Can you work these out from the drawing? Everything is in mm from the part's minimum corner. A direction names the side the tool comes from. Give positions to 0.01 mm unless a question says otherwise; leave off trailing zeros. Write each loop counter-clockwise with the first axis right and the second up, starting at its lowest first coordinate (ties: lowest second). Pieces come first, ordered by that corner, then holes. Notation, with made-up numbers: (89, -8) - (135, -8) arc R21 ccw to (135, 18) - close; hole circle Ø6 at (47.25, 7.25). An arc over 180 degrees is marked (long way). Answer in a Markdown table with one row per item.
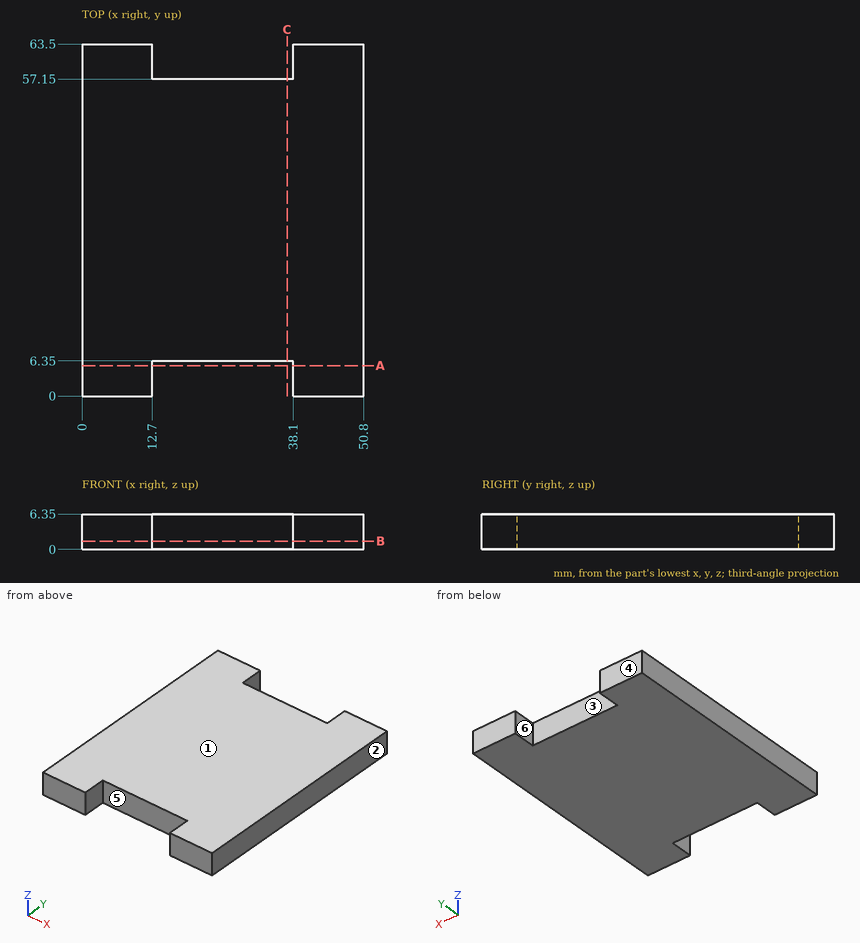
1) We'd pull the mould along X, two halves only. Please class the marked faces 1, 2 and 3: +X half, -X half, draft (parallel to the pull), parting line (faces both ways), or undercut.
Check values:
| item | result |
|---|---|
| face 1 | draft |
| face 2 | +X half |
| face 3 | undercut |
2) Will these pins go through, and if not, where does the flat tip stop? P1, Ø3, axis at x = 33.5, z = 4.5, coming from the +Y side; P2, Ø3, axis at x = 30.5, z = 3.5, coming from the -Y side.
Check values:
| item | result |
|---|---|
| P1 | stops at y = 57.15 |
| P2 | stops at y = 6.35 |
3) Imagine slicing it at A-A (y = 5.5). List the corners of the cut face in (x, z) for me, then the cut area to 3 significant figures.
Check values:
| item | result |
|---|---|
| outline | (0, 0) - (12.7, 0) - (12.7, 6.35) - (0, 6.35) - close; (38.1, 0) - (50.8, 0) - (50.8, 6.35) - (38.1, 6.35) - close |
| area | 161 mm2 |
4) If I drill on line 1 (X direction, y = 59, z = 1); line 2 (Y direction, x = 38, z = 1), over which ranges is the centre line in solid material (lowest first)?
Check values:
| item | result |
|---|---|
| line 1 | x = 0 to 12.7, 38.1 to 50.8 |
| line 2 | y = 6.35 to 57.15 |
5) Imagine slicing it at C-C (x = 37). List the corners of the cut face in (y, z) for me.
Check values:
| item | result |
|---|---|
| outline | (6.35, 0) - (57.15, 0) - (57.15, 6.35) - (6.35, 6.35) - close |
6) On a 3-axis mill with a long thin cutter (end or side, diameter ignored), from which of +Z, -Z, +X, -X, +Y, -Y can I reach the whole of each face in a straight line? I mean the marked faces 4, 5 and 6. Say none if no direction works.
Check values:
| item | result |
|---|---|
| face 4 | +Z, -Z, +X, -X, +Y |
| face 5 | +Z, -Z, -Y |
| face 6 | +Z, -Z, +Y |
7) Imagine slicing it at B-B (z = 1.5). List the corners of the cut face in (x, y) for me.
Check values:
| item | result |
|---|---|
| outline | (0, 0) - (12.7, 0) - (12.7, 6.35) - (38.1, 6.35) - (38.1, 0) - (50.8, 0) - (50.8, 63.5) - (38.1, 63.5) - (38.1, 57.15) - (12.7, 57.15) - (12.7, 63.5) - (0, 63.5) - close |
